Check sheet for the modelled part. Datum: model origin and axes. Units: mm. Face numbers are marked on the shaded views. Give positions to 0.01 mm unless a question says otherwise; leave off trailing zeros. Loops run counter-clockwise (first coordinate to the right, second up) from the corner with the lowest first, then second, coordinate; pieces in that order, holes last.
```python
from build123d import *

# Parameters (mm, degrees)
SKETCH_1_W          = 65
SKETCH_1_H          = 25
SKETCH_1_R          = 3
EXTRUDE_1_DEPTH     = 10
SKETCH_2_R          = 1.5
CUT_EXTRUDE_1_DEPTH = 10


with BuildPart() as part:
    # 草图1 → 凸台-拉伸1 (new body)
    with BuildSketch(Plane(origin=(0, 0, 0), x_dir=(1, 0, 0), z_dir=(0, 1, 0))):
        Rectangle(SKETCH_1_W, SKETCH_1_H)
        with Locations(Location((-10.625, 0, 0), (0, 0, 270))):
            Circle(SKETCH_1_R, mode=Mode.SUBTRACT)
        with Locations(Location((10.625, 0, 0), (0, 0, 270))):
            Circle(SKETCH_1_R, mode=Mode.SUBTRACT)
    extrude(amount=EXTRUDE_1_DEPTH)

    # 草图2 → 切除-拉伸1 (cut)
    with BuildSketch(Plane.XZ):
        with Locations(Location((-26, 10, 0), (0, 0, 270))):
            Circle(SKETCH_2_R)
        with Locations(Location((26, 10, 0), (0, 0, 270))):
            Circle(SKETCH_2_R)
    extrude(amount=-CUT_EXTRUDE_1_DEPTH, mode=Mode.SUBTRACT)


solid = part.part
```
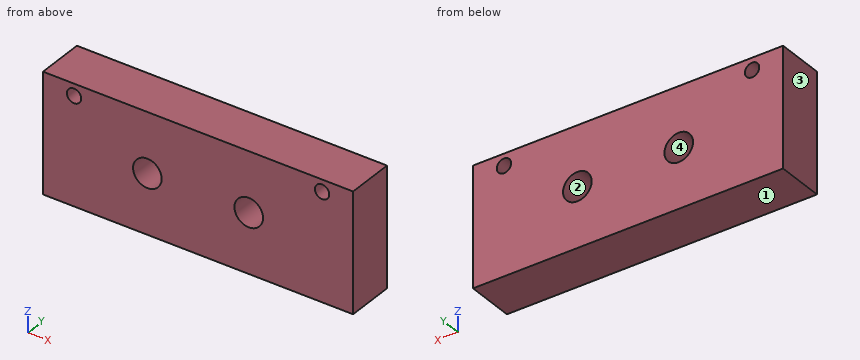
(1) Section check A-A on x = 26. Record the boundary of the cut face in (y, z).
(2) Release check for a two-part mould opening along X. For the marked faces 1, 2, 3 and 4 record: pulls with the +X half, pulls with the -X half, needs draft (parallel to the pull), parting line crosses it, or undercut.
(3) Section check D-D on z = 10. Record the boundary of the cut face in (x, y).
(4) Section check B-B on z = 0. Record the boundary of the cut face in (x, y) (3 decimals).
(5) Section check C-C on y = 7.75. Record the boundary of the cut face in (x, z) (3 decimals), plus the area to 3 significant figures.
(6) Material ranges on line 1 (X direction, y = 5.75, z = 0) (3 decimals); line 2 (X direction, y = 2.75, z = 10); line 3 (Z direction, x = 12, y = 5.5), recorded low to high.
Computed values:
1. outline: (0, -12.5) - (10, -12.5) - (10, 8.5) - (0, 8.5) - close; (0, 11.5) - (10, 11.5) - (10, 12.5) - (0, 12.5) - close
2. face 1: needs draft
2. face 2: undercut
2. face 3: pulls with the -X half
2. face 4: undercut
3. outline: (-32.5, 0) - (-27.5, 0) - (-27.5, 10) - (-32.5, 10) - close; (-24.5, 0) - (24.5, 0) - (24.5, 10) - (-24.5, 10) - close; (27.5, 0) - (32.5, 0) - (32.5, 10) - (27.5, 10) - close
4. outline: (-32.5, 0) - (-13.625, 0) - (-13.625, 10) - (-32.5, 10) - close; (-7.625, 0) - (7.625, 0) - (7.625, 10) - (-7.625, 10) - close; (13.625, 0) - (32.5, 0) - (32.5, 10) - (13.625, 10) - close
5. outline: (-32.5, -12.5) - (32.5, -12.5) - (32.5, 12.5) - (-32.5, 12.5) - close; hole circle Ø3 at (-26, 10); hole circle Ø6 at (-10.625, 0); hole circle Ø6 at (10.625, 0); hole circle Ø3 at (26, 10)
5. area: 1,550 mm2
6. line 1: x = -32.5 to -13.625, -7.625 to 7.625, 13.625 to 32.5
6. line 2: x = -32.5 to -27.5, -24.5 to 24.5, 27.5 to 32.5
6. line 3: z = -12.5 to -2.67, 2.67 to 12.5
